from build123d import *

# Parameters (mm, degrees)
SKETCH1_R           = 3.765
BOSS_EXTRUDE1_DEPTH = 1.78
SKETCH2_R           = 6
SKETCH2_R_2         = 3.765
BOSS_EXTRUDE2_DEPTH = 7


with BuildPart() as part:
    # Sketch1 → Boss-Extrude1 (new body)
    with BuildSketch(Plane.XY):
        with BuildLine():
            Line((-17.975, 14.404110755), (-12.177560595, 8.60667135))
            ThreePointArc((-12.177560595, 8.60667135), (-8.612560595, 0), (-12.177560595, -8.60667135))
            Line((-12.177560595, -8.60667135), (-17.975, -14.404110755))
            ThreePointArc((-17.975, -14.404110755), (-18.714555378, -16.189555378), (-17.975, -17.975))
            ThreePointArc((-17.975, -17.975), (-16.189555378, -18.714555378), (-14.404110755, -17.975))
            Line((-14.404110755, -17.975), (-8.60667135, -12.177560595))
            ThreePointArc((-8.60667135, -12.177560595), (0, -8.612560595), (8.60667135, -12.177560595))
            Line((8.60667135, -12.177560595), (14.404110755, -17.975))
            ThreePointArc((14.404110755, -17.975), (16.189555378, -18.714555378), (17.975, -17.975))
            ThreePointArc((17.975, -17.975), (18.714555378, -16.189555378), (17.975, -14.404110755))
            Line((17.975, -14.404110755), (12.177560595, -8.60667135))
            ThreePointArc((12.177560595, -8.60667135), (8.612560595, 0), (12.177560595, 8.60667135))
            Line((12.177560595, 8.60667135), (17.975, 14.404110755))
            ThreePointArc((17.975, 14.404110755), (18.714555378, 16.189555378), (17.975, 17.975))
            ThreePointArc((17.975, 17.975), (16.189555378, 18.714555378), (14.404110755, 17.975))
            Line((14.404110755, 17.975), (8.60667135, 12.177560595))
            ThreePointArc((8.60667135, 12.177560595), (0, 8.612560595), (-8.60667135, 12.177560595))
            Line((-8.60667135, 12.177560595), (-14.404110755, 17.975))
            ThreePointArc((-14.404110755, 17.975), (-16.189555378, 18.714555378), (-17.975, 17.975))
            ThreePointArc((-17.975, 17.975), (-18.714555378, 16.189555378), (-17.975, 14.404110755))
        make_face()
        Circle(SKETCH1_R, mode=Mode.SUBTRACT)
        with BuildLine():
            ThreePointArc((-17.07, 17.07), (-17.07, 15.599217895), (-15.599217895, 15.599217895))
            ThreePointArc((-15.599217895, 15.599217895), (-15.599217895, 17.07), (-17.07, 17.07))
        make_face(mode=Mode.SUBTRACT)
        with BuildLine():
            ThreePointArc((-15.599217895, -15.599217895), (-17.07, -15.599217895), (-17.07, -17.07))
            ThreePointArc((-17.07, -17.07), (-15.599217895, -17.07), (-15.599217895, -15.599217895))
        make_face(mode=Mode.SUBTRACT)
        with BuildLine():
            ThreePointArc((17.07, 17.07), (15.599217895, 17.07), (15.599217895, 15.599217895))
            ThreePointArc((15.599217895, 15.599217895), (17.07, 15.599217895), (17.07, 17.07))
        make_face(mode=Mode.SUBTRACT)
        with BuildLine():
            ThreePointArc((17.07, -17.07), (17.07, -15.599217895), (15.599217895, -15.599217895))
            ThreePointArc((15.599217895, -15.599217895), (15.599217895, -17.07), (17.07, -17.07))
        make_face(mode=Mode.SUBTRACT)
    extrude(amount=BOSS_EXTRUDE1_DEPTH)

    # Sketch2 → Boss-Extrude2 (add)
    with BuildSketch(Plane.XY.offset(1.78)):
        Circle(SKETCH2_R)
        Circle(SKETCH2_R_2, mode=Mode.SUBTRACT)
    extrude(amount=BOSS_EXTRUDE2_DEPTH)


solid = part.part
Input: part model. Units: mm. Frame: model coordinates. A direction names the side the tool comes from. Coordinates: 2 decimals unless noted, no trailing zeros. Loops run counter-clockwise (first coordinate to the right, second up) from the corner with the lowest first, then second, coordinate; pieces in that order, holes last. Notation, with made-up numbers: (-13.5, -20) - (-9.5, -20) arc R27 ccw to (-9.5, 19) - close; hole circle Ø10 at (50, 79). An arc over 180 degrees is marked (long way). Answer in a Markdown table with one row per item. Add a question column.
Item 1: Contact query for flat-ended pins moving along their axis: P1, Ø4, axis at x = 14, z = 5.5, coming from the +Y side; P2, Ø5, axis at x = 11.5, y = -7, coming from the +Z side; P3, Ø1.5, axis at x = 4, z = 1, coming from the -Y side; P4, Ø3.5, axis at x = -16.33, y = -16.33, coming from the -Z side. Output: stop coordinate, or through.
Item 2: Section query C-C on y = 5. Return the cut outline in (x, z), then the cut area to 3 significant figures.
Item 3: Section query A-A on y = 0. Return the cut outline in (x, z) (3 decimals), then the cut area to 3 significant figures.
Item 4: Line query: line 1 along Z through (x, y) = (3.5, 6); line 2 along X through (y, z) = (-14.5, 0.75); line 3 along Y through (x, z) = (-2, 1). Output: solid intervals per line, ascending. Write a range as [from, to].
Item 5: Mould query, pull axis Y, two halves, no side actions, for faces 4 (the flat face through (15.036, 11.465, 0.878)), 5 (the cylindrical face through (-0.134, -8.613, 0.878)), 6 (the cylindrical face through (0.134, 8.613, 0.878)). Classes: released by +Y, released by -Y, zero draft, split by the parting line, or undercut.
Item 6: Section query D-D on z = 7.25. Return the cut outline in (x, y) (3 decimals), then the cut area to 3 significant figures.
Item 7: Access query for faces 1 (the cylindrical face through (-6, 0, 5)), 2 (the flat face through (11.465, -15.036, 0.878)), 3 (the flat face through (-15.12, 11.55, 0.88)). Directions: +Z, -Z, +X, -X, +Y, -Y. A direction counts if a zero-diameter tool reaches every point of the face in a straight line with its end or side. Return the directions, or none.
Recorded:
| question | item | result |
|---|---|---|
| 1 | P1 | through |
| 1 | P2 | z = 1.78 |
| 1 | P3 | y = -9.58 |
| 1 | P4 | z = 0 |
| 2 | outline | (-9.69, 0) - (9.69, 0) - (9.69, 1.78) - (3.32, 1.78) - (3.32, 8.78) - (-3.32, 8.78) - (-3.32, 1.78) - (-9.69, 1.78) - close |
| 2 | area | 80.9 mm^2 |
| 3 | outline | (-8.613, 0) - (-3.765, 0) - (-3.765, 8.78) - (-6, 8.78) - (-6, 1.78) - (-8.613, 1.78) - close; (3.765, 0) - (8.613, 0) - (8.613, 1.78) - (6, 1.78) - (6, 8.78) - (3.765, 8.78) - close |
| 3 | area | 48.5 mm^2 |
| 4 | line 1 | [0, 1.78] |
| 4 | line 2 | [-18.07, -10.93], [10.93, 18.07] |
| 4 | line 3 | [-8.78, -3.19], [3.19, 8.78] |
| 5 | face 4 | undercut |
| 5 | face 5 | released by -Y |
| 5 | face 6 | released by +Y |
| 6 | outline | circle Ø12 at (0, 0); hole circle Ø7.53 at (0, 0) |
| 6 | area | 68.6 mm^2 |
| 7 | face 1 | +Z |
| 7 | face 2 | +Z, -Z, -Y |
| 7 | face 3 | +Z, -Z, -X |
